Geometry: see drawing. Coordinates: mm, zero at the bounding-box minimum. Coordinates: 2 decimals unless noted, no trailing zeros. Loops run counter-clockwise (first coordinate to the right, second up) from the corner with the lowest first, then second, coordinate; pieces in that order, holes last. Notation, with made-up numbers: M -39.75,64.25 L -16.75,64.25 A37 ccw -16.75,101.25 Z; hole C 31,78.5 d8. An arc over 180 degrees is marked long. One line per question, with ' | ' between items. Start each with the question number.
1. Section query C-C, the plane y = 6.25. Output: boundary loops of the cut face in (x, z), and give its area (3 significant figures).
2. Ray query, probe 1 along X at (y, z) = (0.75, 10.5); probe 2 along Z at (x, y) = (8.5, 2.5); probe 3 along X at (y, z) = (5, 20). Return the intervals inside material, ascending.
3. Pin query (flat end, axial travel): P1, Ø1.8, axis at x = 21, y = 4.5, coming from the +Z side; P2, Ø3, axis at x = 35.5, y = 4, coming from the -Z side; P3, Ø1.8, axis at y = 5.5, z = 32.5, coming from the -X side. Return the tip coordinate at first contact, or that it passes through.
4. Section query B-B, the plane x = 16. Output: boundary loops of the cut face in (y, z).
5. Mould query, pull axis X, two halves, no side actions, for the marked faces 1 and 2. Classes: pulls with the +X half, pulls with the -X half, needs draft (parallel to the pull), parting line crosses it, or undercut.
6. Section query A-A, the plane z = 23. Output: boundary loops of the cut face in (x, y).
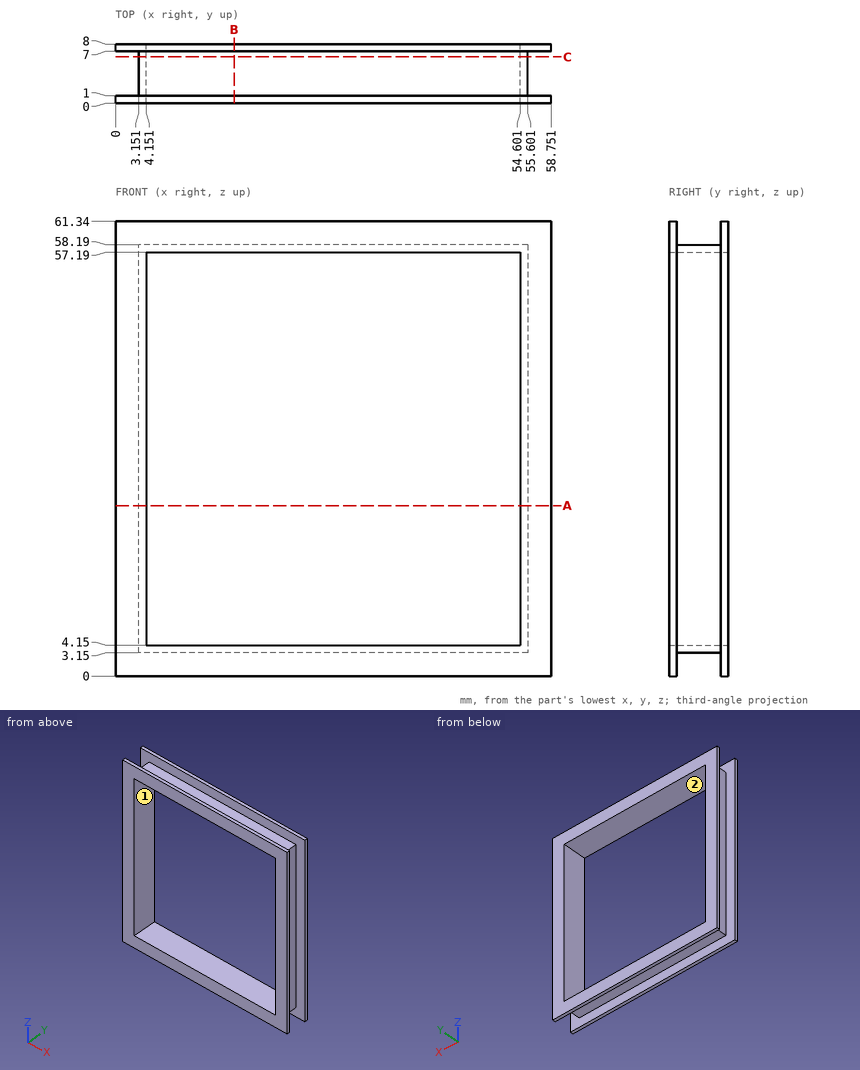
Taken from the geometry:
1) outline: M 3.15,3.15 L 55.6,3.15 L 55.6,58.19 L 3.15,58.19 Z; hole M 4.15,4.15 L 54.6,4.15 L 54.6,57.19 L 4.15,57.19 Z | area: 211 mm^2
2) probe 1: 0 to 4.15, 54.6 to 58.75 | probe 2: 3.15 to 4.15, 57.19 to 58.19 | probe 3: 3.15 to 4.15, 54.6 to 55.6
3) P1: z = 58.19 | P2: z = 3.15 | P3: x = 3.15
4) outline: M 0,0 L 1,0 L 1,3.15 L 7,3.15 L 7,0 L 8,0 L 8,4.15 L 0,4.15 Z; M 0,57.19 L 8,57.19 L 8,61.34 L 7,61.34 L 7,58.19 L 1,58.19 L 1,61.34 L 0,61.34 Z
5) face 1: undercut | face 2: undercut
6) outline: M 0,0 L 4.15,0 L 4.15,8 L 0,8 L 0,7 L 3.15,7 L 3.15,1 L 0,1 Z; M 54.6,0 L 58.75,0 L 58.75,1 L 55.6,1 L 55.6,7 L 58.75,7 L 58.75,8 L 54.6,8 Z
